Check sheet for the drawn part. Datum: minimum x, y, z corner. Units: mm. Give positions to 0.01 mm unless a question says otherwise; leave off trailing zeros. Loops run counter-clockwise (first coordinate to the right, second up) from the corner with the lowest first, then second, coordinate; pieces in that order, holes last.
1. Cross-section at B-B, the plane x = 7.25. Record the cut outline in (y, z), plus the area to 3 significant figures.
2. Cross-section at C-C, the plane z = 0.8. Record the cut outline in (x, y) (3 decimals), plus the area to 3 significant figures.
3. Go/stop test with flat-tipped pins: pin 1 Ø4 at (x, y) = (11.445, 10.21) entering from +Z; pin 2 Ø1 at (x, z) = (6.5, 2.5) entering from +Y; pin 3 Ø1.3 at (y, z) = (6, 2.5) entering from +X. Record where each tip stops, or that it passes through.
4. Cross-section at D-D, the plane y = 7. Record the cut outline in (x, z).
5. Cross-section at A-A, the plane y = 10.21. Record the cut outline in (x, z) (3 decimals), plus the area to 3 significant figures.
6. Release check for a two-part mould opening along Y. For the marked faces 1, 2, 3 and 4 record: +Y half, -Y half, draft (parallel to the pull), parting line (faces both ways), or undercut.
7. Material ranges on L1, parallel to Z at x = 9.25, y = 4.25; L2, parallel to Y at x = 3, z = 0.1; L3, parallel to Y at x = 6, z = 2.2, recorded low to high.
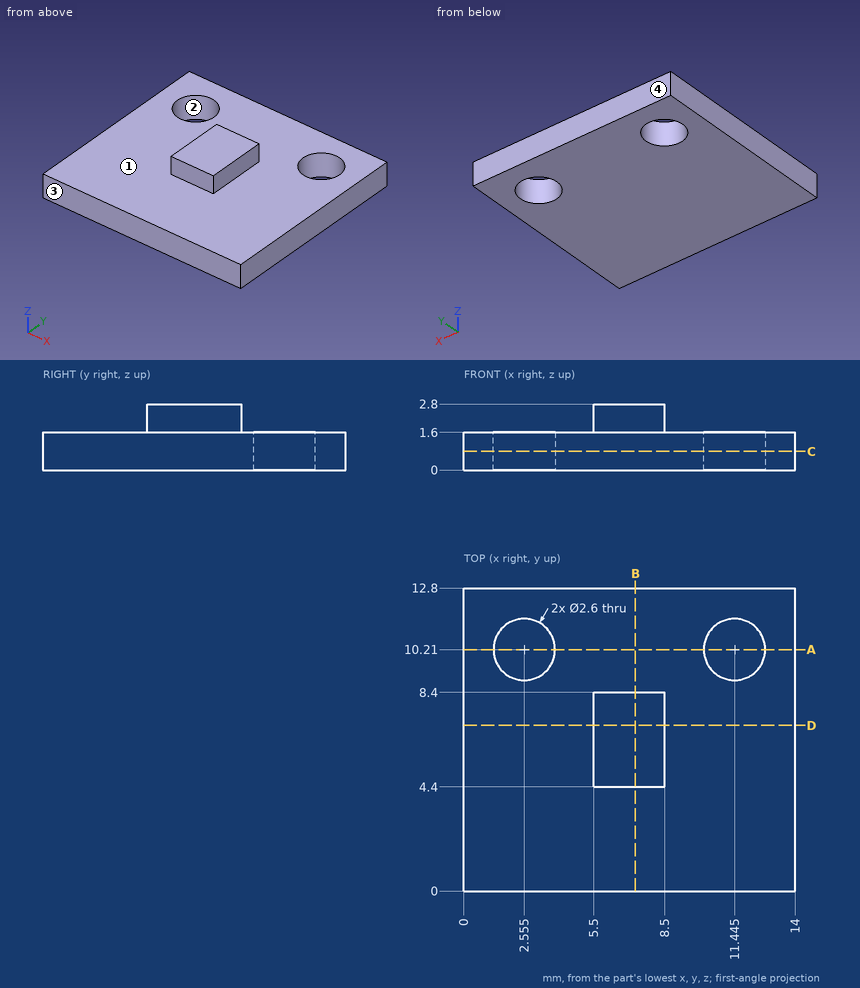
Result:
1. outline: (0, 0) - (12.8, 0) - (12.8, 1.6) - (8.4, 1.6) - (8.4, 2.8) - (4.4, 2.8) - (4.4, 1.6) - (0, 1.6) - close
1. area: 25.3 mm2
2. outline: (0, 0) - (14, 0) - (14, 12.8) - (0, 12.8) - close; hole circle Ø2.6 at (2.555, 10.21); hole circle Ø2.6 at (11.445, 10.21)
2. area: 169 mm2
3. pin 1: stops at z = 1.6
3. pin 2: stops at y = 8.4
3. pin 3: stops at x = 8.5
4. outline: (0, 0) - (14, 0) - (14, 1.6) - (8.5, 1.6) - (8.5, 2.8) - (5.5, 2.8) - (5.5, 1.6) - (0, 1.6) - close
5. outline: (0, 0) - (1.255, 0) - (1.255, 1.6) - (0, 1.6) - close; (3.855, 0) - (10.145, 0) - (10.145, 1.6) - (3.855, 1.6) - close; (12.745, 0) - (14, 0) - (14, 1.6) - (12.745, 1.6) - close
5. area: 14.1 mm2
6. face 1: draft
6. face 2: undercut
6. face 3: -Y half
6. face 4: +Y half
7. L1: z = 0 to 1.6
7. L2: y = 0 to 8.99, 11.43 to 12.8
7. L3: y = 4.4 to 8.4
